```python
from build123d import *

# Parameters (mm, degrees)
SKETCH1_W           = 15
SKETCH1_H           = 20.25
BOSS_EXTRUDE1_DEPTH = 1.6
SKETCH2_W           = 2.5
SKETCH2_H           = 20.25
BOSS_EXTRUDE2_DEPTH = 2.5
SKETCH3_W           = 9
SKETCH3_H           = 9
BOSS_EXTRUDE3_DEPTH = 6
CUT_EXTRUDE1_REACH  = 16.25
SKETCH4_W           = 1
SKETCH4_H           = 3.5


with BuildPart() as part:
    # Sketch1 → Boss-Extrude1 (new body)
    with BuildSketch(Plane(origin=(0, 0, 0), x_dir=(1, 0, 0), z_dir=(0, 1, 0))):
        with Locations((7.5, 10.125)):
            Rectangle(SKETCH1_W, SKETCH1_H)
    extrude(amount=BOSS_EXTRUDE1_DEPTH)

    # Sketch2 → Boss-Extrude2 (add)
    with BuildSketch(Plane.XZ):
        with Locations((1.25, -10.125)):
            Rectangle(SKETCH2_W, SKETCH2_H)
        with Locations((13.75, -10.125)):
            Rectangle(SKETCH2_W, SKETCH2_H)
    extrude(amount=BOSS_EXTRUDE2_DEPTH)

    # Sketch3 → Boss-Extrude3 (add)
    with BuildSketch(Plane(origin=(0, 1.6, 0), x_dir=(1, 0, 0), z_dir=(0, 1, 0))):
        with Locations((7, 10.5)):
            Rectangle(SKETCH3_W, SKETCH3_H)
    extrude(amount=BOSS_EXTRUDE3_DEPTH)

    # Sketch4 → Cut-Extrude1 (cut, up to next)
    with BuildSketch(Plane.XY.offset(-6), mode=Mode.PRIVATE) as cut_extrude1_sk1:
        with Locations((4, 5.85)):
            Rectangle(SKETCH4_W, SKETCH4_H)
    cut_extrude1_tool1 = extrude(cut_extrude1_sk1.sketch, amount=-CUT_EXTRUDE1_REACH, mode=Mode.PRIVATE) & part.part
    add(cut_extrude1_tool1.solids().sort_by_distance((4, 5.85, -6))[0], mode=Mode.SUBTRACT)
    # Sketch4 → Cut-Extrude1 (cut, up to next)
    with BuildSketch(Plane.XY.offset(-6), mode=Mode.PRIVATE) as cut_extrude1_sk2:
        with Locations((6, 5.85)):
            Rectangle(SKETCH4_W, SKETCH4_H)
    cut_extrude1_tool2 = extrude(cut_extrude1_sk2.sketch, amount=-CUT_EXTRUDE1_REACH, mode=Mode.PRIVATE) & part.part
    add(cut_extrude1_tool2.solids().sort_by_distance((6, 5.85, -6))[0], mode=Mode.SUBTRACT)
    # Sketch4 → Cut-Extrude1 (cut, up to next)
    with BuildSketch(Plane.XY.offset(-6), mode=Mode.PRIVATE) as cut_extrude1_sk3:
        with Locations((8, 5.85)):
            Rectangle(SKETCH4_W, SKETCH4_H)
    cut_extrude1_tool3 = extrude(cut_extrude1_sk3.sketch, amount=-CUT_EXTRUDE1_REACH, mode=Mode.PRIVATE) & part.part
    add(cut_extrude1_tool3.solids().sort_by_distance((8, 5.85, -6))[0], mode=Mode.SUBTRACT)
    # Sketch4 → Cut-Extrude1 (cut, up to next)
    with BuildSketch(Plane.XY.offset(-6), mode=Mode.PRIVATE) as cut_extrude1_sk4:
        with Locations((10, 5.85)):
            Rectangle(SKETCH4_W, SKETCH4_H)
    cut_extrude1_tool4 = extrude(cut_extrude1_sk4.sketch, amount=-CUT_EXTRUDE1_REACH, mode=Mode.PRIVATE) & part.part
    add(cut_extrude1_tool4.solids().sort_by_distance((10, 5.85, -6))[0], mode=Mode.SUBTRACT)


solid = part.part
```
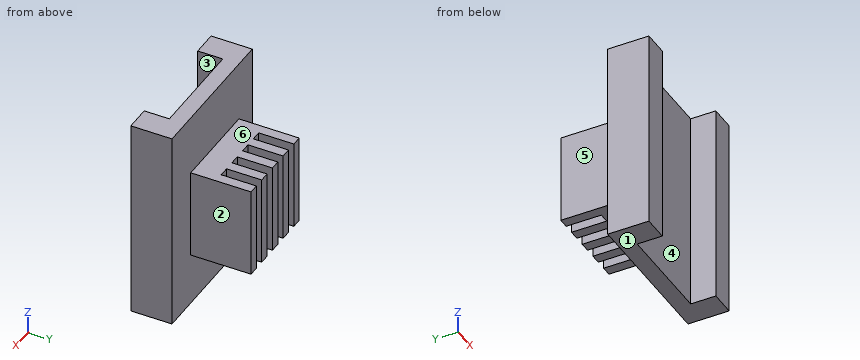
CAD build for the part. Positions are in the model's coordinates, mm. Face numbers are marked on the shaded views. A direction names the side the tool comes from. Coordinates: 2 decimals unless noted, no trailing zeros. Order: outer loops, then holes, each group sorted by start corner. A loop starts at its lowest first (then second) coordinate and runs counter-clockwise, first axis right, second up. Notation, with made-up numbers: M 84.5,-22 L 126.5,-22 A17 cw 126.5,-6 Z; hole C -37,10.5 d4. An arc over 180 degrees is marked long. Write each question's results on one line, items separated by ' | '. Start each with the question number.
Q1. Cut at A-A (y = -0.5). List the corners of the cut face in (x, z), then the cut area to 3 significant figures.
Q2. Cut at D-D (z = -8). List the corners of the cut face in (x, y).
Q3. Which spindle directions (+Z, -Z, +X, -X, +Y, -Y) get a long thin tool onto all of the face, cutting with end or side? Do the marked faces 4, 5 and 6. Say none if no direction does.
Q4. Pull direction X, two halves, no side cores. Call the marked faces 1, 2 and 3: +X half, -X half, draft (parallel to the pull), parting line (faces both ways), or undercut.
Q5. Cut at C-C (y = 6.5). List the corners of the cut face in (x, z), then the cut area to 3 significant figures.
Q6. Cut at B-B (x = 11). List the corners of the cut face in (y, z), then the cut area to 3 significant figures.
Q7. Flat gauge pins, fed straight in: P1, Ø6, axis at x = 8, z = -16, coming from the -Y side; P2, Ø1.8, axis at y = 6.5, z = -12, coming from the -X side; P3, Ø4, axis at y = 6.5, z = -8.5, coming from the +X side. Where does each tip first touch, or does it go through?
Q8. Drill centre lines: probe 1 along X at (y, z) = (5.25, -12); probe 2 along X at (y, z) = (-0.25, -7); probe 3 along Y at (x, z) = (11.25, -12.75). Where is each one in solid material? Low to high. Write a range as from..to.
Found:
1) outline: M 0,-20.25 L 2.5,-20.25 L 2.5,0 L 0,0 Z; M 12.5,-20.25 L 15,-20.25 L 15,0 L 12.5,0 Z | area: 101 mm²
2) outline: M 0,-2.5 L 2.5,-2.5 L 2.5,0 L 12.5,0 L 12.5,-2.5 L 15,-2.5 L 15,1.6 L 11.5,1.6 L 11.5,7.6 L 10.5,7.6 L 10.5,4.1 L 9.5,4.1 L 9.5,7.6 L 8.5,7.6 L 8.5,4.1 L 7.5,4.1 L 7.5,7.6 L 6.5,7.6 L 6.5,4.1 L 5.5,4.1 L 5.5,7.6 L 4.5,7.6 L 4.5,4.1 L 3.5,4.1 L 3.5,7.6 L 2.5,7.6 L 2.5,1.6 L 0,1.6 Z
3) face 4: +Z, -Z, -Y | face 5: +Z, -Z, -X, +Y | face 6: +Z, +X, -X, +Y
4) face 1: draft | face 2: +X half | face 3: undercut
5) outline: M 2.5,-15 L 3.5,-15 L 3.5,-6 L 2.5,-6 Z; M 4.5,-15 L 5.5,-15 L 5.5,-6 L 4.5,-6 Z; M 6.5,-15 L 7.5,-15 L 7.5,-6 L 6.5,-6 Z; M 8.5,-15 L 9.5,-15 L 9.5,-6 L 8.5,-6 Z; M 10.5,-15 L 11.5,-15 L 11.5,-6 L 10.5,-6 Z | area: 45.0 mm²
6) outline: M 0,-20.25 L 1.6,-20.25 L 1.6,-15 L 7.6,-15 L 7.6,-6 L 1.6,-6 L 1.6,0 L 0,0 Z | area: 86.4 mm²
7) P1: y = 0 | P2: x = 2.5 | P3: x = 11.5
8) probe 1: 2.5..3.5, 4.5..5.5, 6.5..7.5, 8.5..9.5, 10.5..11.5 | probe 2: 0..2.5, 12.5..15 | probe 3: 0..7.6
